```python
from build123d import *

# Parameters (mm, degrees)
SCHIZZO1_R                   = 45
ESTRUSIONE_ESTRUSIONE1_DEPTH = 2
CROQUIS1_R                   = 2
CROQUIS1_W                   = 40.7
CROQUIS1_H                   = 20
CORTAR_EXTRUIR1_DEPTH        = 10


with BuildPart() as part:
    # Schizzo1 → Estrusione-Estrusione1 (new body, symmetric)
    with BuildSketch(Plane(origin=(0, 0, 0), x_dir=(1, 0, 0), z_dir=(0, 1, 0))):
        Circle(SCHIZZO1_R)
    extrude(amount=ESTRUSIONE_ESTRUSIONE1_DEPTH, both=True)

    # Croquis1 → Cortar-Extruir1 (cut)
    with BuildSketch(Plane(origin=(0, 2, 0), x_dir=(1, 0, 0), z_dir=(0, 1, 0))):
        with Locations((-34.7, 5)):
            Circle(CROQUIS1_R)
        with Locations((-34.7, -5)):
            Circle(CROQUIS1_R)
        with Locations((0, -21.25)):
            Circle(CROQUIS1_R)
        with Locations((0, 21.25)):
            Circle(CROQUIS1_R)
        with Locations((14, 5)):
            Circle(CROQUIS1_R)
        with Locations((14, -5)):
            Circle(CROQUIS1_R)
        with Locations((-10.35, 0)):
            Rectangle(CROQUIS1_W, CROQUIS1_H)
    extrude(amount=-CORTAR_EXTRUIR1_DEPTH, mode=Mode.SUBTRACT)


solid = part.part
```
Read the model definition and answer for the solid it produces. Units are mm, in the model's axes. A direction names the side the tool comes from. Coordinates: 2 decimals unless noted, no trailing zeros. Loops run counter-clockwise (first coordinate to the right, second up) from the corner with the lowest first, then second, coordinate; pieces in that order, holes last.
(1) A tool of negligible diameter and unlimited length cuts with its end or side. For faces 4 (the face through (10, 0, 0)), 5 (the face through (-1, -2, -11)), from which of +Z, -Z, +X, -X, +Y, -Y can it reach the whole face along a straight path? Write none if from no direction.
Solution:
face 4: +Y, -Y
face 5: +Z, -Z, +X, -X, -Y
(2) Consider line 1 along Z through (x, y) = (0, 0.8); line 2 along X through (y, z) = (0.2, 5); line 3 along Z through (x, y) = (-34.7, -0.95). Determine where each line is inside the solid, lowest interval first.
Solution:
line 1: z = -45 to -23.25, -19.25 to -10, 10 to 19.25, 23.25 to 45
line 2: x = -44.72 to -36.7, -32.7 to -30.7, 10 to 12, 16 to 44.72
line 3: z = -28.65 to -7, -3 to 3, 7 to 28.65
(3) Flat-ended cylindrical pins translate along their axes: pin 1 Ø1 at (x, y) = (-35, 1.5) entering from -Z; pin 2 Ø1.5 at (y, z) = (-1, -19.5) entering from +X; pin 3 Ø1.5 at (y, z) = (0, 18) entering from -X; pin 4 Ø8 at (x, z) = (-35.5, -28.5) entering from -Y. Find the tip coordinate at first contact, or state that the pin passes through.
Solution:
pin 1: stops at z = -28.89
pin 2: stops at x = 40.91
pin 3: stops at x = -41.56
pin 4: stops at y = -2
(4) The part is cut by section C-C (y = -0.1). Determine the outline of the cut face in (x, z), and give its area (3 significant figures).
Solution:
outline: circle Ø90 at (0, 0); hole circle Ø4 at (-34.7, -5); hole circle Ø4 at (-34.7, 5); hole (-30.7, -10) - (10, -10) - (10, 10) - (-30.7, 10) - close; hole circle Ø4 at (0, -21.25); hole circle Ø4 at (0, 21.25); hole circle Ø4 at (14, -5); hole circle Ø4 at (14, 5)
area: 5,470 mm2
(5) The part is cut by section A-A (z = 0). Determine the outline of the cut face in (x, y).
Solution:
outline: (-45, -2) - (-30.7, -2) - (-30.7, 2) - (-45, 2) - close; (10, -2) - (45, -2) - (45, 2) - (10, 2) - close
(6) The part is cut by section B-B (x = 0). Determine the outline of the cut face in (y, z), and give its area (3 significant figures).
Solution:
outline: (-2, -45) - (2, -45) - (2, -23.25) - (-2, -23.25) - close; (-2, -19.25) - (2, -19.25) - (2, -10) - (-2, -10) - close; (-2, 10) - (2, 10) - (2, 19.25) - (-2, 19.25) - close; (-2, 23.25) - (2, 23.25) - (2, 45) - (-2, 45) - close
area: 248 mm2
(7) The mould has two halves that part along Z. Classify faces 1 (the face through (20.765, 0.028, 39.923)), 2 (the face through (-32.853, 0.028, 5.766)), 3 (the face through (-1, 2, -11)): released by +Z, released by -Z, zero draft, split by the parting line, or undercut.
Solution:
face 1: split by the parting line
face 2: undercut
face 3: zero draft
(8) The part is cut by section D-D (x = -12). Determine the outline of the cut face in (y, z), and give its area (3 significant figures).
Solution:
outline: (-2, -43.37) - (2, -43.37) - (2, -10) - (-2, -10) - close; (-2, 10) - (2, 10) - (2, 43.37) - (-2, 43.37) - close
area: 267 mm2
